Model file for the job. Use its own axes, mm. Face numbers are marked on the shaded views. A direction names the side the tool comes from. Coordinates: 2 decimals unless noted, no trailing zeros. Write each loop counter-clockwise with the first axis right and the second up, starting at its lowest first coordinate (ties: lowest second). Pieces come first, ordered by that corner, then holes.
Q1. Drill centre lines: probe 1 along X at (y, z) = (-0.5, 0); probe 2 along Y at (x, z) = (-1, -1); probe 3 along X at (y, z) = (1.75, -1). Where is each one in solid material? Low to high.
Q2. Band-saw the part on B-B, the plane y = 4.5. Write the cut outline in (x, z).
Q3. Which spindle directions (+Z, -Z, +X, -X, +Y, -Y) get a long thin tool onto all of the face, cutting with end or side? Do the marked faces 1, 2, 3, 4 and 5. Say none if no direction does.
Q4. Band-saw the part on A-A, the plane z = -3.2. State how many separate pieces and enclosed holes the cut face has, plus the area to 3 significant figures.
Q5. Pin check, flat tips, straight feed: P1, Ø0.8, axis at x = -2, z = 3.5, coming from the -Y side; P2, Ø1.9, axis at x = -2, z = 4, coming from the +Y side; P3, Ø5, axis at y = 0, z = 3.5, coming from the +X side. Stop position of each tip, or through.
Q6. Pull direction Z, two halves, no side cores. Call the marked faces 6, 7 and 8: released by +Z, released by -Z, zero draft, split by the parting line, or undercut.
from build123d import *

# Parameters (mm, degrees)
SKETCH3_R           = 1.2
CUT_EXTRUDE1_DEPTH  = 6
BOSS_EXTRUDE1_START = -0.01
BOSS_EXTRUDE1_DEPTH = 2
CIRPATTERN1_COUNT   = 12
CHAMFER1_SIZE       = 0.3
SKETCH6_W           = 0.5
SKETCH6_H           = 14.8
SKETCH7_W           = 1.6
SKETCH7_H           = 0.6
SKETCH8_W           = 1.8
SKETCH8_H           = 1.5
SKETCH9_R           = 4.9
BOSS_EXTRUDE2_DEPTH = 2.09


with BuildPart() as part:
    # Sketch2 → Revolve1 (revolve)
    with BuildSketch(Plane(origin=(0, 0, 0), x_dir=(0, 0, -1), z_dir=(1, 0, 0))):
        Polygon((0, 2.1), (4.9, 2.1), (4.9, -2.1), (5.25, -2.1), (5.25, 2.9), (0, 2.9), align=None)
    revolve(axis=Axis((0, -2.1, 0), (0, 1, 0)))

    # Sketch3 → Cut-Extrude1 (cut, through all)
    with BuildSketch(Plane(origin=(0, 2.9, 0), x_dir=(1, 0, 0), z_dir=(0, 1, 0))):
        with Locations((0, 3.2)):
            Circle(SKETCH3_R)
        with Locations((3.043380852, 0.988854382)):
            Circle(SKETCH3_R)
        with Locations((1.880912807, -2.588854382)):
            Circle(SKETCH3_R)
        with Locations((-1.880912807, -2.588854382)):
            Circle(SKETCH3_R)
        with Locations((-3.043380852, 0.988854382)):
            Circle(SKETCH3_R)
    extrude(amount=-CUT_EXTRUDE1_DEPTH, mode=Mode.SUBTRACT)

    # Sketch4 → Boss-Extrude1 (add)
    with BuildSketch(Plane.XZ.offset(2.1).offset(BOSS_EXTRUDE1_START)):
        with BuildLine():
            Line((1.064115017, -4.114627472), (1.22686202, -4.743923438))
            ThreePointArc((1.22686202, -4.743923438), (0, -4.9), (-1.22686202, -4.743923438))
            Line((-1.22686202, -4.743923438), (-1.064115017, -4.114627472))
            ThreePointArc((-1.064115017, -4.114627472), (0, -4.25), (1.064115017, -4.114627472))
        make_face()
    boss_extrude1 = extrude(amount=-BOSS_EXTRUDE1_DEPTH)

    # CirPattern1: Boss-Extrude1 ×12 about axis
    cirpattern1_axis = Axis((0, 0, 0), (0, 1, 0))
    for i in range(1, CIRPATTERN1_COUNT):
        add(boss_extrude1.rotate(cirpattern1_axis, i * 360 / CIRPATTERN1_COUNT))

    # Chamfer1
    chamfer1_edges = [part.edges().sort_by_distance(p)[0] for p in [
        (0, 2.9, 5.25),
    ]]
    chamfer(chamfer1_edges, length=CHAMFER1_SIZE)

    # Sketch6 → Revolve2 (revolve)
    with BuildSketch(Plane.XY):
        with Locations((0.25, 1.3)):
            Rectangle(SKETCH6_W, SKETCH6_H)
    revolve(axis=Axis((0, -6.1, 0), (0, 1, 0)))

    # Sketch7 → Revolve3 (revolve)
    with BuildSketch(Plane.XY):
        Polygon((0, 2.9), (1.6, 2.9), (1.6, 3.2), (0.75, 3.2), (0.75, 3.65), (0.5, 3.9), (0, 3.9), (0, 3.2), align=None)
        with Locations((0.8, -5.1)):
            Rectangle(SKETCH7_W, SKETCH7_H)
    revolve(axis=Axis((0, 3.2, 0), (0, 1, 0)))

    # Sketch8 → Revolve4 (revolve)
    with BuildSketch(Plane.XY):
        with Locations((0.9, 1.35)):
            Rectangle(SKETCH8_W, SKETCH8_H)
    revolve(axis=Axis((0, 2.1, 0), (0, -1, 0)))

    # Sketch9 → Boss-Extrude2 (add)
    with BuildSketch(Plane.XZ.offset(-2.1)):
        Circle(SKETCH9_R)
        with BuildLine():
            ThreePointArc((2.586255154, 3.559674743), (3.920428719, 1.997558174), (4.4, 0))
            ThreePointArc((4.4, 0), (4.345828698, -0.688311651), (4.184648669, -1.359674785))
            ThreePointArc((4.184648669, -1.359674785), (2.586255106, -3.559674778), (-1e-09, -4.4))
            ThreePointArc((-1e-09, -4.4), (-2.586255112, -3.559674774), (-4.184648673, -1.359674772))
            ThreePointArc((-4.184648673, -1.359674772), (-4.184648682, 1.359674743), (-2.586255168, 3.559674733))
            ThreePointArc((-2.586255168, 3.559674733), (-8e-09, 4.4), (2.586255154, 3.559674743))
        make_face(mode=Mode.SUBTRACT)
    extrude(amount=BOSS_EXTRUDE2_DEPTH)


solid = part.part
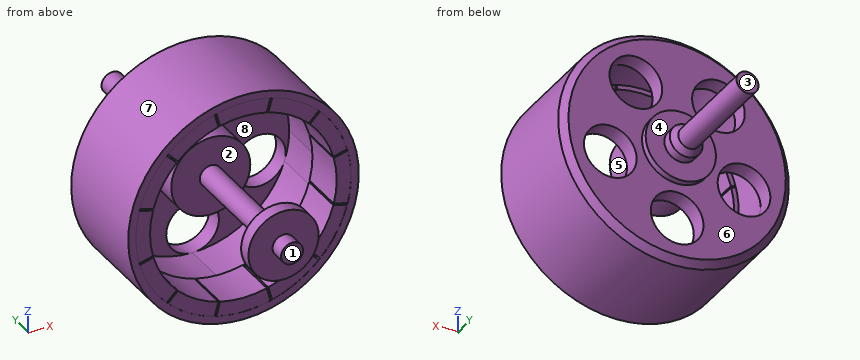
Answer sheet:
1. probe 1: x = -5.25 to -4.25, -0.5 to 0.5, 4.25 to 5.25
1. probe 2: y = -5.4 to -4.8, 0.6 to 3.2
1. probe 3: x = -5.15 to -4.28, -1.5 to 1.5, 4.28 to 5.15
2. outline: circle Ø1 at (0, 0)
3. face 1: +Z, -Z, +X, -X, -Y
3. face 2: none
3. face 3: +Z, -Z, +X, -X, +Y
3. face 4: +Y
3. face 5: -Y
4. separate pieces: 4
4. enclosed holes: 0
4. area: 14.5 mm2
5. P1: stops at y = -2.09
5. P2: stops at y = 2.9
5. P3: stops at x = 5.15
6. face 6: zero draft
6. face 7: split by the parting line
6. face 8: undercut
